from build123d import *

# Parameters (mm, degrees)
SKETCH1_W           = 467.2
SKETCH1_H           = 222.25
BOSS_EXTRUDE1_DEPTH = 5
SKETCH2_W           = 467.2
SKETCH2_H           = 462.2
BOSS_EXTRUDE2_DEPTH = 5
SKETCH3_W           = 287.2
SKETCH3_H           = 674.4
CUT_EXTRUDE1_DEPTH  = 165


with BuildPart() as part:
    # Sketch1 → Boss-Extrude1 (new body)
    with BuildSketch(Plane.XY):
        Rectangle(SKETCH1_W, SKETCH1_H)
    extrude(amount=BOSS_EXTRUDE1_DEPTH)

    # Sketch2 → Boss-Extrude2 (add)
    with BuildSketch(Plane(origin=(0, 111.125, 0), x_dir=(1, 0, 0), z_dir=(0, 1, 0))):
        with Locations((0, 226.1)):
            Rectangle(SKETCH2_W, SKETCH2_H)
    extrude(amount=BOSS_EXTRUDE2_DEPTH)

    # Sketch3 → Cut-Extrude1 (cut)
    with BuildSketch(Plane(origin=(0, 116.125, 0), x_dir=(1, 0, 0), z_dir=(0, 1, 0))):
        with Locations((0, -5)):
            Rectangle(SKETCH3_W, SKETCH3_H)
    extrude(amount=-CUT_EXTRUDE1_DEPTH, mode=Mode.SUBTRACT)


solid = part.part
Build history of the part. All positions in model axes, mm. A direction names the side the tool comes from. Coordinates: 2 decimals unless noted, no trailing zeros. Order: outer loops, then holes, each group sorted by start corner. A loop starts at its lowest first (then second) coordinate and runs counter-clockwise, first axis right, second up. Notation, with made-up numbers: (35.25, 78.5) - (66.25, 78.5) arc R28 cw to (66.25, 114.5) - close; hole circle Ø1 at (-12, 35.5). An arc over 180 degrees is marked (long way). Put each result on its own line as item: value.
1. Saw through at D-D (z = -360). Write the cut outline in (x, y) (3 decimals), and give its area (3 significant figures).
Answer sheet:
outline: (-233.6, 111.125) - (233.6, 111.125) - (233.6, 116.125) - (-233.6, 116.125) - close
area: 2,340 mm^2
2. Saw through at B-B (z = -141.5). Write the cut outline in (x, y) (3 decimals).
Answer sheet:
outline: (-233.6, 111.125) - (-143.6, 111.125) - (-143.6, 116.125) - (-233.6, 116.125) - close; (143.6, 111.125) - (233.6, 111.125) - (233.6, 116.125) - (143.6, 116.125) - close
3. Saw through at C-C (x = 164). Write the cut outline in (y, z) (3 decimals).
Answer sheet:
outline: (-111.125, 0) - (111.125, 0) - (111.125, -457.2) - (116.125, -457.2) - (116.125, 5) - (-111.125, 5) - close
4. Probe line 1 along Z through (x, y) = (-23, -87); line 2 along Y through (x, z) = (93.5, -438.5) (3 decimals). List the from-to ranges inside material, lowest first. Write a range as [from, to].
Answer sheet:
line 1: z = [0, 5]
line 2: y = [111.125, 116.125]
5. Drop flat-ended pins along their axis: P1, Ø3, axis at x = -175, z = -292.5, coming from the -Y side (3 decimals); P2, Ø1.5, axis at x = 24, z = 1.5, coming from the +Y side (3 decimals); P3, Ø4, axis at x = -45.5, y = 113.5, coming from the +Z side. Give the stop position or say it passes through.
Answer sheet:
P1: stops at y = 111.125
P2: stops at y = -48.875
P3: stops at z = -332.2
6. Saw through at A-A (y = 82). Write the cut outline in (x, z).
Answer sheet:
outline: (-233.6, 0) - (-143.6, 0) - (-143.6, 5) - (-233.6, 5) - close; (143.6, 0) - (233.6, 0) - (233.6, 5) - (143.6, 5) - close
7. Tool access for faces 1 (the face through (-3, 111.125, -333)), 2 (the face through (233.6, 111.4, -225)): list every direction of +Z, -Z, +X, -X, +Y, -Y with a clear straight run to the whole face (end or side of a thin tool).
Answer sheet:
face 1: -Z, +X, -X, -Y
face 2: +Z, -Z, +X, +Y, -Y
